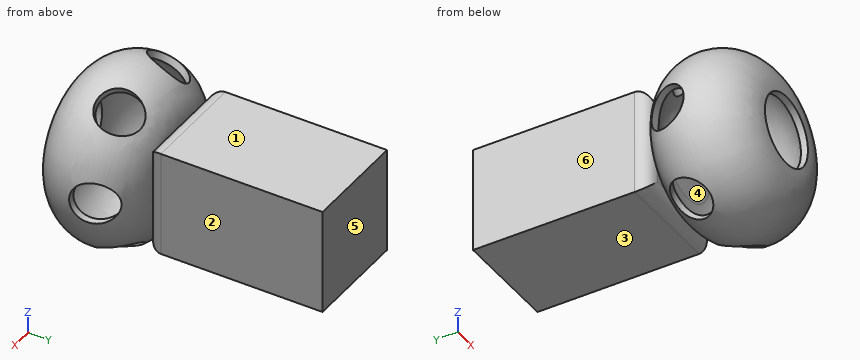
```python
from build123d import *

# Parameters (mm, degrees)
SKETCH3_R           = 1.5
CUT_EXTRUDE1_DEPTH  = 12.592023292
CIRPATTERN1_COUNT   = 6
SKETCH4_W           = 7.5
SKETCH4_H           = 7.5
BOSS_EXTRUDE2_DEPTH = 12.5
FILLET1_R           = 1


with BuildPart() as part:
    # Sketch2 → Revolve1 (revolve)
    with BuildSketch(Plane.XY, mode=Mode.PRIVATE) as revolve1_sk:
        with BuildLine():
            Line((2.5, 7.5), (0, 7.5))
            Line((0, 7.5), (0, 7))
            Line((0, 7), (2.5, 7))
            ThreePointArc((2.5, 7), (5.75, 3.75), (2.5, 0.5))
            Line((2.5, 0.5), (2.5, 0))
            ThreePointArc((2.5, 0), (6.25, 3.75), (2.5, 7.5))
        make_face()
    revolve(revolve1_sk.sketch.rotate(Axis((0, 0, 0), (0, 1, 0)), 90), axis=Axis((0, 0, 0), (0, 1, 0)))

    # Sketch3 → Cut-Extrude1 (cut, symmetric)
    with BuildSketch(Plane(origin=(0, 0, 0), x_dir=(0, 0, -1), z_dir=(1, 0, 0))):
        with Locations(Location((0, 5, 0), (0, 0, 75.140884096))):
            Circle(SKETCH3_R)
    cut_extrude1 = extrude(amount=CUT_EXTRUDE1_DEPTH, both=True, mode=Mode.SUBTRACT)

    # CirPattern1: Cut-Extrude1 ×6 about axis
    cirpattern1_axis = Axis((0, 0, 0), (0, 1, 0))
    for i in range(1, CIRPATTERN1_COUNT):
        add(cut_extrude1.rotate(cirpattern1_axis, i * 360 / CIRPATTERN1_COUNT), mode=Mode.SUBTRACT)

    # Sketch4 → Boss-Extrude2 (add)
    with BuildSketch(Plane(origin=(0, 7.5, 0), x_dir=(1, 0, 0), z_dir=(0, 1, 0))):
        Rectangle(SKETCH4_W, SKETCH4_H)
    extrude(amount=BOSS_EXTRUDE2_DEPTH)

    # Fillet1
    fillet1_edges = [part.edges().sort_by_distance(p)[0] for p in [
        (3.75, 7.5, 0),
        (0, 7.5, -3.75),
        (-3.75, 7.5, 0),
        (0, 7.5, 3.75),
    ]]
    fillet(fillet1_edges, radius=FILLET1_R)


solid = part.part
```
Check sheet for the modelled part. Datum: model origin and axes. Units: mm. Face numbers are marked on the shaded views. A direction names the side the tool comes from. Round coordinates to 2 decimals unless told otherwise and drop trailing zeros. Loops run counter-clockwise (first coordinate to the right, second up) from the corner with the lowest first, then second, coordinate; pieces in that order, holes last. Notation, with made-up numbers: (7.25, -29) - (33.25, -29) arc R35 cw to (33.25, 10) - close; hole circle Ø10 at (24.5, 0). An arc over 180 degrees is marked (long way). Write item = value, one per line. Start each with the question number.
Q1. Access from +Z, -Z, +X, -X, +Y, -Y to the whole of each face (thin tool, end or side, straight path). Record for the marked faces 1, 2 and 3.
Q2. Section check A-A (z = 0). Count the separate pieces of the cut face and the enclosed holes in it, plus the area to 3 significant figures.
Q3. Section check B-B (y = 8.75). Record the boundary of the cut face in (x, z).
Q4. Release check for a two-part mould opening along X. For the marked faces 4, 5 and 6 record: pulls with the +X half, pulls with the -X half, needs draft (parallel to the pull), parting line crosses it, or undercut.
Q5. Depth check by flat-ended pin: P1, Ø3, axis at y = 9, z = 5, coming from the +X side; P2, Ø5, axis at y = 5, z = 0, coming from the -X side; P3, Ø2, axis at x = 3, y = 13.5, coming from the +Z side. Enter the tip coordinate at first touch or a pass-through.
Q6. Thickness scan on L1, parallel to X at y = 18.25, z = -3; L2, parallel to Y at x = 1.25, z = 2. Record the ranges inside material, lowest first.
Derived:
q1.face_1 = +Z, +X, -X, +Y
q1.face_2 = +Z, -Z, +X, +Y
q1.face_3 = -Z, +X, -X, +Y
q2.separate_pieces = 3
q2.enclosed_holes = 0
q2.area = 103 mm^2
q3.outline = (-3.75, -3.75) - (3.75, -3.75) - (3.75, 3.75) - (-3.75, 3.75) - close
q4.face_4 = undercut
q4.face_5 = needs draft
q4.face_6 = pulls with the -X half
q5.P1 = 3.75
q5.P2 = -6.24
q5.P3 = 3.75
q6.L1 = -3.75 to 3.75
q6.L2 = 7 to 20
